Work out the finished part from the listing and answer in its coordinate system (mm). Give positions to 0.01 mm unless a question says otherwise; leave off trailing zeros. Loops run counter-clockwise (first coordinate to the right, second up) from the corner with the lowest first, then second, coordinate; pieces in that order, holes last. Notation, with made-up numbers: M 68.5,17.5 L 77.5,17.5 A33 ccw 77.5,46.5 Z; hole C 43,65 d2. An arc over 180 degrees is marked long. Write item = value, one per line. Start each with the question number.
1. The mould has two halves that part along Z. Classify faces 1 (the face through (601, -15, -50.8)), 2 (the face through (601, -15, 0)), 3 (the face through (0, -15, -26)), 4 (the face through (307.946, -15.027, -34.623)): released by +Z, released by -Z, zero draft, split by the parting line, or undercut.
2. Section B-B on y = -18 is taken. Determine the outline of the cut face in (x, z), plus the area to 3 significant figures.
3. Section A-A on x = 320.04 is taken. Determine the outline of the cut face in (y, z), plus the area to 3 significant figures.
4. Consider L1, parallel to X at y = -12.5, z = -26; L2, parallel to X at y = -28, z = -31; L3, parallel to Z at x = 320.04, y = -9. Determine where each line is inside the solid, lowest interval first. Write a range as [from, to].
```python
from build123d import *

# Parameters (mm, degrees)
F0_W     = 1219.2
F0_H     = 50.8
F0_R     = 9.144
F0_R_2   = 15.24
F1_DEPTH = 30.48
F2_DEPTH = 30.48
F3_DEPTH = 30.48
F4_DEPTH = 30.48


with BuildPart() as f1:
    # F0 (on Front) → F1 (new body)
    with BuildSketch(Plane.XZ):
        with Locations((609.6, -25.4)):
            Rectangle(F0_W, F0_H)
        with Locations((25.542894, -25.4508)):
            Circle(F0_R, mode=Mode.SUBTRACT)
        with Locations((320.04, -25.3492)):
            Circle(F0_R_2, mode=Mode.SUBTRACT)
    extrude(amount=F1_DEPTH)

    # F0 (on Front) → F2 (join)
    with BuildSketch(Plane.XZ):
        with Locations((609.6, -25.4)):
            Rectangle(F0_W, F0_H)
        with Locations((25.542894, -25.4508)):
            Circle(F0_R, mode=Mode.SUBTRACT)
        with Locations((320.04, -25.3492)):
            Circle(F0_R_2, mode=Mode.SUBTRACT)
    extrude(amount=F2_DEPTH)

    # F0 (on Front) → F3 (join)
    with BuildSketch(Plane.XZ):
        with Locations((609.6, -25.4)):
            Rectangle(F0_W, F0_H)
        with Locations((25.542894, -25.4508)):
            Circle(F0_R, mode=Mode.SUBTRACT)
        with Locations((320.04, -25.3492)):
            Circle(F0_R_2, mode=Mode.SUBTRACT)
    extrude(amount=F3_DEPTH)

    # F0 (on Front) → F4 (join)
    with BuildSketch(Plane.XZ):
        with Locations((609.6, -25.4)):
            Rectangle(F0_W, F0_H)
        with Locations((25.542894, -25.4508)):
            Circle(F0_R, mode=Mode.SUBTRACT)
        with Locations((320.04, -25.3492)):
            Circle(F0_R_2, mode=Mode.SUBTRACT)
    extrude(amount=F4_DEPTH)


solid = f1.part
```
Verdict:
q1.face_1 = released by -Z
q1.face_2 = released by +Z
q1.face_3 = zero draft
q1.face_4 = undercut
q2.outline = M 0,-50.8 L 1219.2,-50.8 L 1219.2,0 L 0,0 Z; hole C 25.54,-25.45 d18.29; hole C 320.04,-25.35 d30.48
q2.area = 60,900 mm2
q3.outline = M -30.48,-50.8 L 0,-50.8 L 0,-40.59 L -30.48,-40.59 Z; M -30.48,-10.11 L 0,-10.11 L 0,0 L -30.48,0 Z
q3.area = 619 mm2
q4.L1 = [0, 16.42], [34.67, 304.81], [335.27, 1219.2]
q4.L2 = [0, 18.28], [32.81, 305.89], [334.19, 1219.2]
q4.L3 = [-50.8, -40.59], [-10.11, 0]
